Print and shaded views of the part. All mm, measured from the part's lowest x, y and z. A direction names the side the tool comes from. Coordinates: 2 decimals unless noted, no trailing zeros. Order: outer loops, then holes, each group sorted by start corner. A loop starts at its lowest first (then second) coordinate and runs counter-clockwise, first axis right, second up. Notation, with made-up numbers: (-13, 14.25) -> (42, 14.25) arc R18 cw to (42, 21.25) -> close; hole circle Ø5 at (-15, 8.5). An arc over 180 degrees is marked (long way). Use one line per item in the form item = value. Start each with the question number.
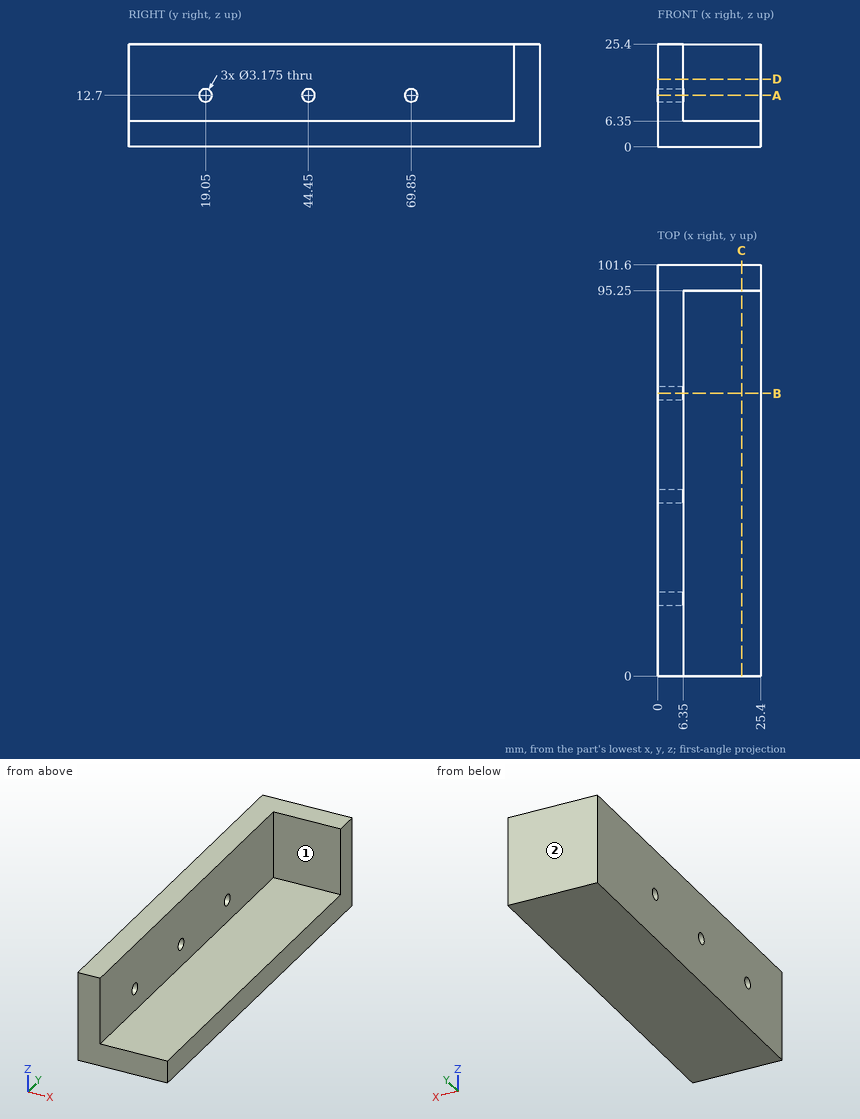
1) 3-axis set-ups, long thin cutter, end or side, ignore diameter. For the marked faces 1 and 2: which of +Z, -Z, +X, -X, +Y, -Y reach the whole face in a straight line?
2) Cut at C-C on x = 20.75. Give the cut face in (y, z), then the cut area to 3 significant figures.
3) Probe L1, parallel to Z at x = 2.75, y = 19.05; L2, parallel to X at y = 25, z = 14.75; L3, parallel to Y at x = 17.5, z = 19.75. List the from-to ranges inside material, lowest first.
4) Cut at D-D on z = 16.75. Give the cut face in (x, y).
5) Drop flat-ended pins along their axis: P1, Ø15, axis at y = 53, z = 19.5, coming from the +X side; P2, Ø1, axis at x = 8.5, z = 22, coming from the -Y side. Give the stop position or say it passes through.
6) Cut at A-A on z = 12.7. Give the cut face in (x, y), then the cut area to 3 significant figures.
7) Cut at B-B on y = 69.85. Give the cut face in (x, z), then the cut area to 3 significant figures.
Values follow:
q1.face_1 = +Z, +X, -Y
q1.face_2 = +Z, -Z, +X, -X, +Y
q2.outline = (0, 0) -> (101.6, 0) -> (101.6, 25.4) -> (95.25, 25.4) -> (95.25, 6.35) -> (0, 6.35) -> close
q2.area = 766 mm^2
q3.L1 = 0 to 11.11, 14.29 to 25.4
q3.L2 = 0 to 6.35
q3.L3 = 95.25 to 101.6
q4.outline = (0, 0) -> (6.35, 0) -> (6.35, 95.25) -> (25.4, 95.25) -> (25.4, 101.6) -> (0, 101.6) -> close
q5.P1 = 6.35
q5.P2 = 95.25
q6.outline = (0, 0) -> (6.35, 0) -> (6.35, 17.46) -> (0, 17.46) -> close; (0, 20.64) -> (6.35, 20.64) -> (6.35, 42.86) -> (0, 42.86) -> close; (0, 46.04) -> (6.35, 46.04) -> (6.35, 68.26) -> (0, 68.26) -> close; (0, 71.44) -> (6.35, 71.44) -> (6.35, 95.25) -> (25.4, 95.25) -> (25.4, 101.6) -> (0, 101.6) -> close
q6.area = 706 mm^2
q7.outline = (0, 0) -> (25.4, 0) -> (25.4, 6.35) -> (6.35, 6.35) -> (6.35, 11.11) -> (0, 11.11) -> close; (0, 14.29) -> (6.35, 14.29) -> (6.35, 25.4) -> (0, 25.4) -> close
q7.area = 262 mm^2
